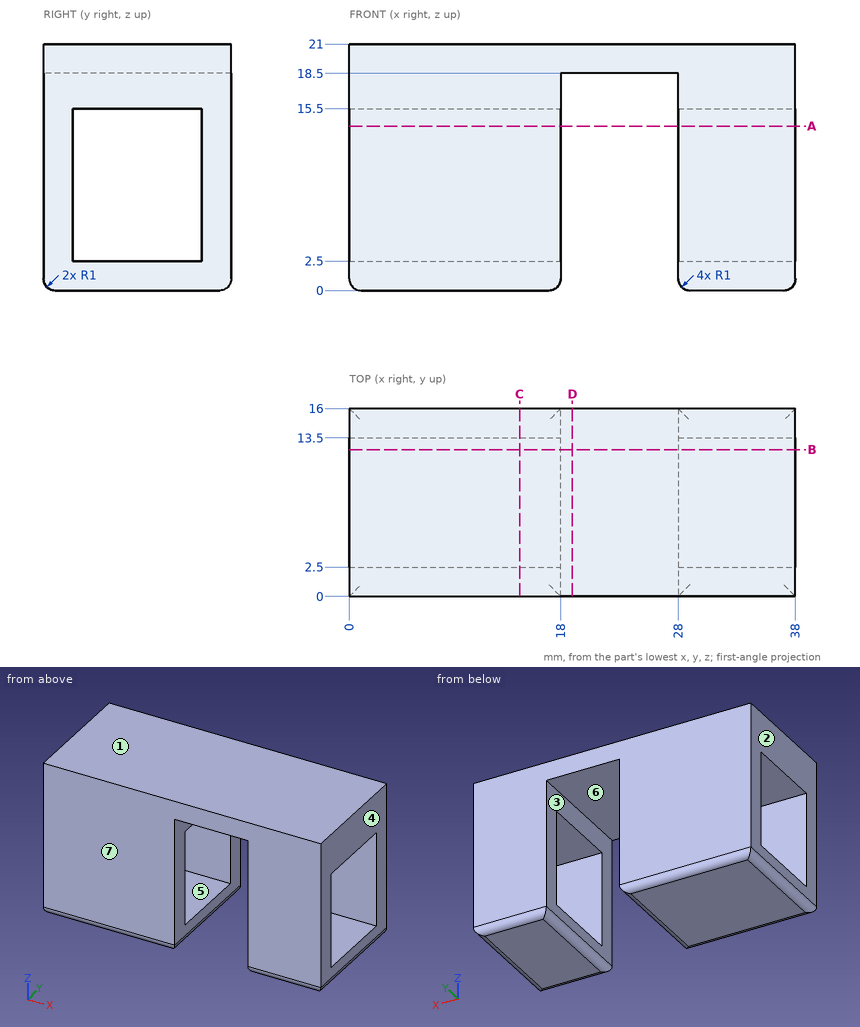
Verification items for this drawing (mm, ordinates from the low corner). A direction names the side the tool comes from. Round coordinates to 2 decimals unless told otherwise and drop trailing zeros. Order: outer loops, then holes, each group sorted by start corner. A loop starts at its lowest first (then second) coordinate and runs counter-clockwise, first axis right, second up.
1) Cross-section at C-C, the plane x = 14.5. Record the cut outline in (y, z), plus the area to 3 significant figures.
Geometry says:
outline: (0, 1) arc R1 ccw to (1, 0) - (15, 0) arc R1 ccw to (16, 1) - (16, 21) - (0, 21) - close; hole (2.5, 2.5) - (13.5, 2.5) - (13.5, 15.5) - (2.5, 15.5) - close
area: 193 mm2
2) Tool access check on the marked faces 5, 6 and 7. Record the directions out of +Z, -Z, +X, -X, +Y, -Y that give a thin tool (end or side, any length) a straight path to the whole face; none if there is none.
Geometry says:
face 5: +X, -X
face 6: -Z, +Y, -Y
face 7: +Z, -Z, +X, -X, -Y
3) Cross-section at A-A, the plane z = 14. Record the cut outline in (x, y).
Geometry says:
outline: (0, 0) - (18, 0) - (18, 2.5) - (0, 2.5) - close; (0, 13.5) - (18, 13.5) - (18, 16) - (0, 16) - close; (28, 0) - (38, 0) - (38, 2.5) - (28, 2.5) - close; (28, 13.5) - (38, 13.5) - (38, 16) - (28, 16) - close
4) Cross-section at D-D, the plane x = 19. Record the cut outline in (y, z).
Geometry says:
outline: (0, 18.5) - (16, 18.5) - (16, 21) - (0, 21) - close
5) Depth check by flat-ended pin: pin 1 (5 mm diameter, centred on y = 7, z = 12, fed in from -X) (3 decimals); pin 2 (5 mm diameter, centred on x = 24, y = 8.5, fed in from -Z). Enter the tip coordinate at first touch or a pass-through.
Geometry says:
pin 1: passes through
pin 2: stops at z = 18.5
6) Draft check along X on the marked faces 1, 2, 3 and 4. Enter one of: +X half, -X half, draft (parallel to the pull), parting line (faces both ways), or undercut.
Geometry says:
face 1: draft
face 2: -X half
face 3: undercut
face 4: +X half
7) Material ranges on line 1 (Y direction, x = 29.5, z = 8.25); line 2 (X direction, y = 11.75, z = 2); line 3 (Z direction, x = 6, y = 12.5), recorded low to high.
Geometry says:
line 1: y = 0 to 2.5, 13.5 to 16
line 2: x = 0 to 18, 28 to 38
line 3: z = 0 to 2.5, 15.5 to 21
8) Cross-section at B-B, the plane y = 12.5. Record the cut outline in (x, z), plus the area to 3 significant figures.
Geometry says:
outline: (0, 1) arc R1 ccw to (1, 0) - (17, 0) arc R1 ccw to (18, 1) - (18, 2.5) - (0, 2.5) - close; (0, 15.5) - (18, 15.5) - (18, 18.5) - (28, 18.5) - (28, 15.5) - (38, 15.5) - (38, 21) - (0, 21) - close; (28, 1) arc R1 ccw to (29, 0) - (37, 0) arc R1 ccw to (38, 1) - (38, 2.5) - (28, 2.5) - close
area: 248 mm2
